from build123d import *

# Parameters (mm, degrees)
RESSALTO_EXTRUS_O1_DEPTH = 10
ESBO_O3_R                = 2
CORTE_EXTRUS_O1_DEPTH    = 15
CHANFRO1_SIZE            = 1.6
FILETE1_R                = 0.5
CHANFRO5_SIZE            = 2
CHANFRO8_SIZE            = 1
ESBO_O4_R                = 1.65
CORTE_EXTRUS_O2_DEPTH    = 10
FILETE2_R                = 0.5
ESBO_O5_R                = 1.65
CORTE_EXTRUS_O3_DEPTH    = 10
FILETE3_R                = 0.5


with BuildPart() as part:
    # Esboço1 → Ressalto-extrusão1 (new body)
    with BuildSketch(Plane.XY):
        Polygon((-0.113617837, 14.25), (-6.113617837, 14.25), (-6.113617837, -0.95), (13.886382163, -0.95), (13.886382163, -5.95), (-6.113617837, -5.95), (-6.113617837, -20.95), (-11.113617837, -20.95), (-11.113617837, 14.25), (-41.113617837, 14.25), (-41.113617837, 19.25), (-0.113617837, 19.25), align=None)
    extrude(amount=RESSALTO_EXTRUS_O1_DEPTH)

    # Esboço3 → Corte-extrusão1 (cut)
    with BuildSketch(Plane.XZ.offset(5.95)):
        with Locations(Location((5.886382163, 5, 0), (0, 0, 270))):
            Circle(ESBO_O3_R)
    extrude(amount=-CORTE_EXTRUS_O1_DEPTH, mode=Mode.SUBTRACT)

    # Chanfro1
    chanfro1_edges = [part.edges().sort_by_distance(p)[0] for p in [
        (5.886382163, -5.95, 7),
    ]]
    chamfer(chanfro1_edges, length=CHANFRO1_SIZE)

    # Filete1
    filete1_edges = [part.edges().sort_by_distance(p)[0] for p in [
        (5.886382163, -0.95, 7),
    ]]
    fillet(filete1_edges, radius=FILETE1_R)

    # Chanfro5
    chanfro5_edges = [part.edges().sort_by_distance(p)[0] for p in [
        (13.886382163, -5.95, 5),
        (-11.113617837, 14.25, 5),
        (-0.113617837, 19.25, 5),
    ]]
    chamfer(chanfro5_edges, length=CHANFRO5_SIZE)

    # Chanfro8
    chanfro8_edges = [part.edges().sort_by_distance(p)[0] for p in [
        (-41.113617837, 19.25, 5),
        (-41.113617837, 16.75, 10),
        (-41.113617837, 14.25, 5),
        (-41.113617837, 16.75, 0),
        (-0.113617837, 15.75, 0),
        (-21.613617837, 19.25, 0),
        (13.886382163, -2.45, 0),
        (12.886382163, -4.95, 0),
        (2.886382163, -5.95, 0),
        (-11.113617837, -4.35, 0),
        (-12.113617837, 13.25, 0),
        (-27.113617837, 14.25, 0),
        (13.886382163, -2.45, 10),
        (12.886382163, -4.95, 10),
        (2.886382163, -5.95, 10),
        (-11.113617837, -4.35, 10),
        (-12.113617837, 13.25, 10),
        (-27.113617837, 14.25, 10),
        (-0.113617837, 15.75, 10),
        (-21.613617837, 19.25, 10),
        (-1.113617837, 18.25, 0),
        (-1.113617837, 18.25, 10),
        (-11.113617837, -20.95, 5),
        (-8.613617837, -20.95, 10),
        (-6.113617837, -13.45, 10),
        (-6.113617837, -20.95, 5),
        (-6.113617837, -13.45, 0),
        (-8.613617837, -20.95, 0),
    ]]
    chamfer(chanfro8_edges, length=CHANFRO8_SIZE)

    # Esboço4 → Corte-extrusão2 (cut)
    with BuildSketch(Plane(origin=(0, 19.25, 0), x_dir=(1, 0, 0), z_dir=(0, 1, 0))):
        with Locations(Location((-35.963617837, -5, 0), (0, 0, 270))):
            Circle(ESBO_O4_R)
    extrude(amount=-CORTE_EXTRUS_O2_DEPTH, mode=Mode.SUBTRACT)

    # Filete2
    filete2_edges = [part.edges().sort_by_distance(p)[0] for p in [
        (-35.963617837, 14.25, 3.35),
        (-35.963617837, 19.25, 3.35),
    ]]
    fillet(filete2_edges, radius=FILETE2_R)

    # Esboço5 → Corte-extrusão3 (cut)
    with BuildSketch(Plane.ZY.offset(11.113617837)):
        with Locations((5, -10.95)):
            Circle(ESBO_O5_R)
    extrude(amount=-CORTE_EXTRUS_O3_DEPTH, mode=Mode.SUBTRACT)

    # Filete3
    filete3_edges = [part.edges().sort_by_distance(p)[0] for p in [
        (-6.113617837, -10.95, 3.35),
        (-11.113617837, -10.95, 3.35),
    ]]
    fillet(filete3_edges, radius=FILETE3_R)


solid = part.part
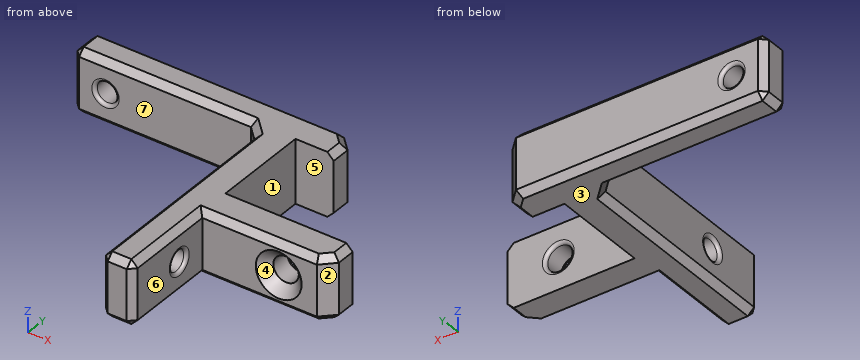
Design review of the part built by this model. Coordinates are the model's own, in mm. Face numbers are marked on the shaded views. A direction names the side the tool comes from. Coordinates: 2 decimals unless noted, no trailing zeros. Loops run counter-clockwise (first coordinate to the right, second up) from the corner with the lowest first, then second, coordinate; pieces in that order, holes last. Notation, with made-up numbers: M 25,-10.5 L 71,-10.5 A26 cw 71,16.5 Z; hole C 86,5 d3. An arc over 180 degrees is marked long. Use one line per item in the form item = value.
(1) Consider section C-C (x = -17.5). Write out the cut boundary in (y, z), and give its area (3 significant figures).
Return value:
outline = M 14.25,1 L 15.25,0 L 18.25,0 L 19.25,1 L 19.25,9 L 18.25,10 L 15.25,10 L 14.25,9 Z
area = 48.0 mm2
(2) For the marked faces 4, 5, 6 and 7, list the 3-axis set-ups (+Z, -Z, +X, -X, +Y, -Y) from which the entire face can be reached by the end or side of a thin tool; tool diameter is ignored.
Return value:
face_4 = -Y
face_5 = +Z, -Z, +X
face_6 = +Z, -Z, +X, -Y
face_7 = +Z, -Z, -X, -Y
(3) Consider section B-B (y = -10.95). Write out the cut boundary in (x, z).
Return value:
outline = M -11.11,1 L -10.11,0 L -7.11,0 L -6.11,1 L -6.11,2.85 A0.5 ccw -6.61,3.35 L -10.61,3.35 A0.5 ccw -11.11,2.85 Z; M -11.11,7.15 A0.5 ccw -10.61,6.65 L -6.61,6.65 A0.5 ccw -6.11,7.15 L -6.11,9 L -7.11,10 L -10.11,10 L -11.11,9 Z
(4) Draft analysis for pull direction Y (two halves, no side actions). For the marked faces 1, 2 and 3, state which applies: pulls with the +Y half, pulls with the -Y half, needs draft (parallel to the pull), parting line crosses it, or undercut.
Return value:
face_1 = undercut
face_2 = pulls with the -Y half
face_3 = needs draft
(5) Clearance check with flat-ended pins moving along their axes: P1, Ø5, axis at x = 4, z = 7.5, coming from the +Y side; P2, Ø2.5, axis at x = 6.5, z = 4, coming from the -Y side; P3, Ø1, axis at y = -5, z = 2, coming from the +X side; P4, Ø3, axis at x = -35.96, z = 5, coming from the -Y side. State where each tip first meets the part, or that it passes through.
Return value:
P1 = -0.95
P2 = -4.77
P3 = 13.34
P4 = through
(6) For line 1 along Y through (x, z) = (-9.6, 5); line 2 along Y through (x, z) = (-3.5, 8.75); line 3 along X through (y, z) = (-2.8, 5), list the stretches that pass through material, from the lowest coordinate up. Write a range as from..to.
Return value:
line_1 = -20.95..-12.6, -9.3..19.25
line_2 = -5.95..-0.95, 14.25..19.25
line_3 = -11.11..3.89, 7.89..13.89
(7) Consider section A-A (x = -8.5). Write out the cut boundary in (y, z), and give its area (3 significant figures).
Return value:
outline = M -20.95,1 L -19.95,0 L 18.25,0 L 19.25,1 L 19.25,9 L 18.25,10 L -19.95,10 L -20.95,9 Z; hole C -10.95,5 d3.3
area = 391 mm2
(8) Consider section D-D (z = 5). Give the number of separate pieces and of enclosed holes in the cut face, and give its area (3 significant figures).
Return value:
separate_pieces = 4
enclosed_holes = 0
area = 421 mm2
